Design review of the part shown in the three views and the two pictorial views. Dimensions are in mm from the part's minimum x, y and z. A direction names the side the tool comes from. Round coordinates to 2 decimals unless told otherwise and drop trailing zeros. Loops run counter-clockwise (first coordinate to the right, second up) from the corner with the lowest first, then second, coordinate; pieces in that order, holes last. Notation, with made-up numbers: (-0.5, 47) -> (18.5, 47) arc R24 ccw to (18.5, 59) -> close; hole circle Ø2 at (56.25, 21). An arc over 180 degrees is marked (long way). Return JSON: item names as keys, results as strings. Group by question number.
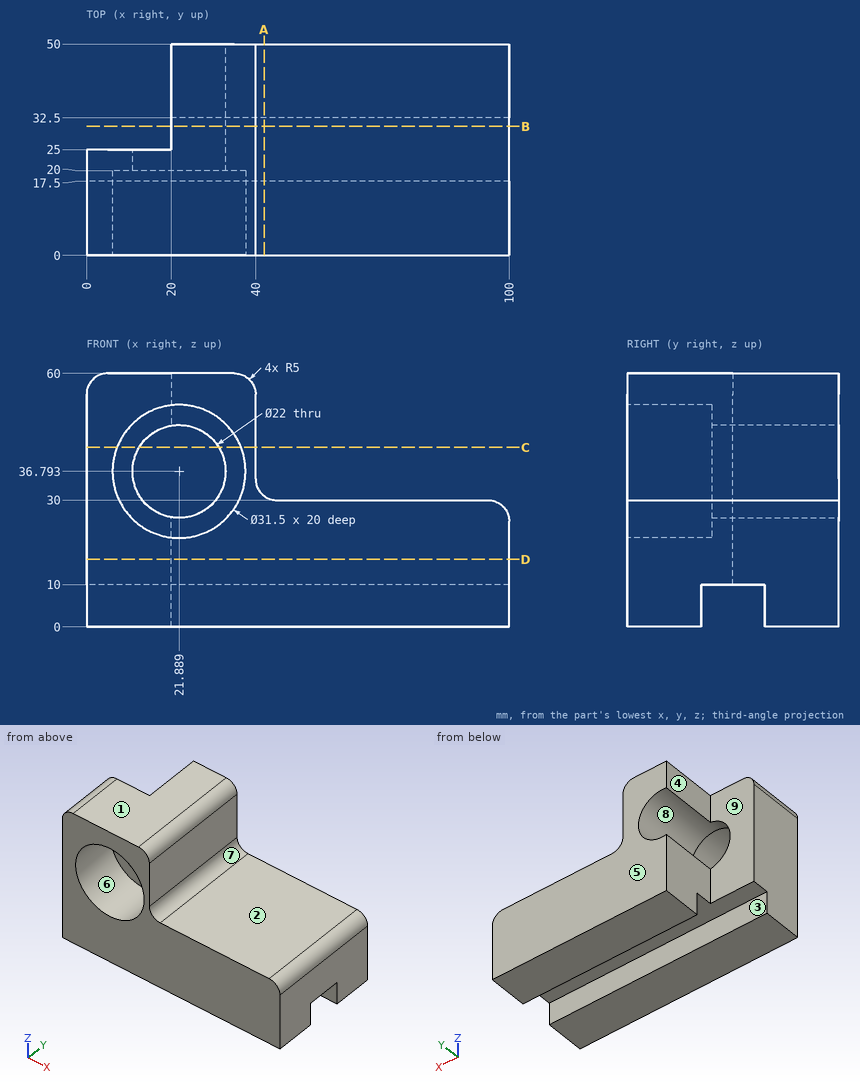
1. Tool access review of the marked faces 1, 2, 3, 4 and 5: name each direction out of +Z, -Z, +X, -X, +Y, -Y from which nothing blocks a thin tool from reaching the whole face with its end or side.
2. Draft analysis for pull direction Z (two halves, no side actions). For the marked faces 6, 7, 8 and 9, state which applies: pulls with the +Z half, pulls with the -Z half, needs draft (parallel to the pull), parting line crosses it, or undercut.
3. We need section A-A, the plane x = 42. Write out the cut boundary in (y, z).
4. We need section B-B, the plane y = 30.5. Write out the cut boundary in (x, z), then the cut area to 3 significant figures.
5. We need section D-D, the plane z = 16. Write out the cut boundary in (x, y), then the cut area to 3 significant figures.
6. For P1, Ø17.5, axis at x = 21.89, z = 36.79, coming from the +Y side; P2, Ø10, axis at x = 5.5, z = 34, coming from the +Y side; P3, Ø16, axis at y = 28.5, z = 43, coming from the +X side; P4, Ø20, axis at y = 42, z = 14.5, coming from the -X side, all flat-tipped, find the tip position at first contact; note any pin that passes through.
7. Wall thickness on line 1 (Y direction, x = 44.5, z = 7); line 2 (Z direction, x = 21, y = 5); line 3 (Z direction, x = 77.5, y = 14.5): over which ranges is each line inside the solid? List them lowest first.
8. We need section C-C, the plane z = 42.5. Write out the cut boundary in (x, y) (1 decimal).
Check sheet entries:
{
 "1": {"face 1": "+Z, +X, -X, +Y, -Y", "face 2": "+Z, +X, +Y, -Y", "face 3": "-Z, +X, -X", "face 4": "+Z, -Z, -X, +Y", "face 5": "+Z, -Z, +X, -X, +Y"},
 "2": {"face 6": "undercut", "face 7": "pulls with the +Z half", "face 8": "undercut", "face 9": "needs draft"},
 "3": {"outline": "(0, 0) -> (17.5, 0) -> (17.5, 10) -> (32.5, 10) -> (32.5, 0) -> (50, 0) -> (50, 31) -> (0, 31) -> close"},
 "4": {"outline": "(20, 10) -> (100, 10) -> (100, 25) arc R5 ccw to (95, 30) -> (45, 30) arc R5 cw to (40, 35) -> (40, 55) arc R5 ccw to (35, 60) -> (20, 60) -> (20, 47.63) arc R11 cw (long way) to (20, 25.96) -> close", "area": "1,960 mm²"},
 "5": {"outline": "(0, 0) -> (100, 0) -> (100, 50) -> (20, 50) -> (20, 25) -> (0, 25) -> close", "area": "4,500 mm²"},
 "6": {"P1": "passes through", "P2": "stops at y = 25", "P3": "stops at x = 40", "P4": "stops at x = 20"},
 "7": {"line 1": "y = 0 to 17.5, 32.5 to 50", "line 2": "z = 0 to 21.07, 52.52 to 60", "line 3": "z = 0 to 30"},
 "8": {"outline": "(0, 0) -> (7.2, 0) -> (7.2, 20) -> (12.5, 20) -> (12.5, 25) -> (0, 25) -> close; (31.3, 20) -> (36.6, 20) -> (36.6, 0) -> (40, 0) -> (40, 50) -> (31.3, 50) -> close"}
}
